Geometry: see drawing. Coordinates: mm, zero at the bounding-box minimum. A direction names the side the tool comes from. Round coordinates to 2 decimals unless told otherwise and drop trailing zeros. Loops run counter-clockwise (first coordinate to the right, second up) from the corner with the lowest first, then second, coordinate; pieces in that order, holes last.
(1) First-contact query: pin 1 Ø1 at (y, z) = (8, 20.5) entering from +X. Flat tip, straight axial feed; report the tip coordinate or a pass-through.
(2) Cut plane B-B, the plane y = 9. Output: boundary loops of the cut face in (x, z).
(3) Line query: line 1 (Y direction, x = 54.5, z = 39); line 2 (X direction, y = 9.25, z = 13.5); line 3 (X direction, y = 11, z = 4). Output: solid intervals per line, ascending.
(4) Draft query along Z for the marked faces 3, 4, 5 and 6. Return one class per face: released by +Z, released by -Z, zero draft, split by the parting line, or undercut.
(5) Access query for the marked faces 1 and 2. Directions: +Z, -Z, +X, -X, +Y, -Y. A direction counts if a zero-diameter tool reaches every point of the face in a straight line with its end or side. Return the directions, or none.
(6) Cut plane A-A, the plane x = 53. Output: boundary loops of the cut face in (y, z).
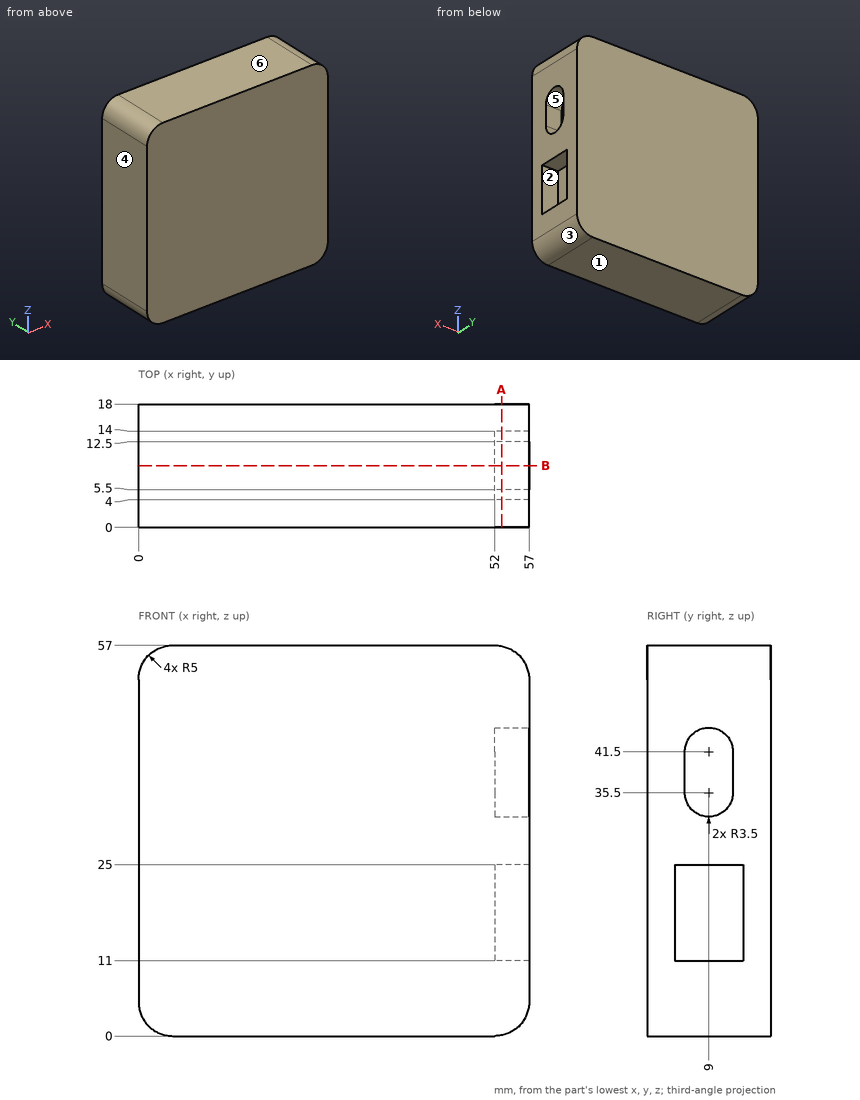
Reported:
1. pin 1: stops at x = 52
2. outline: (0, 5) arc R5 ccw to (5, 0) - (52, 0) arc R5 ccw to (57, 5) - (57, 11) - (52, 11) - (52, 25) - (57, 25) - (57, 32) - (52, 32) - (52, 45) - (57, 45) - (57, 52) arc R5 ccw to (52, 57) - (5, 57) arc R5 ccw to (0, 52) - close
3. line 1: y = 0 to 5.5, 12.5 to 18
3. line 2: x = 0 to 52
3. line 3: x = 0.1 to 56.9
4. face 3: released by -Z
4. face 4: zero draft
4. face 5: undercut
4. face 6: released by +Z
5. face 1: -Z, +X, -X, +Y, -Y
5. face 2: +X
6. outline: (0, 0.1) - (18, 0.1) - (18, 56.9) - (0, 56.9) - close; hole (4, 11) - (14, 11) - (14, 25) - (4, 25) - close; hole (5.5, 35.5) arc R3.5 ccw to (12.5, 35.5) - (12.5, 41.5) arc R3.5 ccw to (5.5, 41.5) - close
